from build123d import *

# Parameters (mm, degrees)
SKETCH_1_R          = 1.5
EXTRUDE_1_DEPTH     = 20
SKETCH_2_R          = 2.5
EXTRUDE_2_DEPTH     = 3
CUT_EXTRUDE_1_DEPTH = 1.5
CHAMFER_1_SIZE      = 0.5


with BuildPart() as part:
    # 草图1 → 凸台-拉伸1 (new body)
    with BuildSketch(Plane.XY):
        Circle(SKETCH_1_R)
    extrude(amount=EXTRUDE_1_DEPTH)

    # 草图2 → 凸台-拉伸2 (add)
    with BuildSketch(Plane.XY.offset(20)):
        Circle(SKETCH_2_R)
    extrude(amount=EXTRUDE_2_DEPTH)

    # 草图3 → 切除-拉伸1 (cut)
    with BuildSketch(Plane.XY.offset(23)):
        Polygon((0, 1.803382283), (-1.56177487, 0.901691141), (-1.56177487, -0.901691141), (0, -1.803382283), (1.56177487, -0.901691141), (1.56177487, 0.901691141), align=None)
    extrude(amount=-CUT_EXTRUDE_1_DEPTH, mode=Mode.SUBTRACT)

    # 倒角1
    chamfer_1_edges = [part.edges().sort_by_distance(p)[0] for p in [
        (-1.5, 0, 0),
    ]]
    chamfer(chamfer_1_edges, length=CHAMFER_1_SIZE)


solid = part.part
Check sheet for the modelled part. Datum: model origin and axes. Units: mm. A direction names the side the tool comes from. Coordinates: 2 decimals unless noted, no trailing zeros. Write each loop counter-clockwise with the first axis right and the second up, starting at its lowest first coordinate (ties: lowest second). Pieces come first, ordered by that corner, then holes.
Item 1: Access from +Z, -Z, +X, -X, +Y, -Y to the whole of each face (thin tool, end or side, straight path). Record for faces 1 (the face through (-1.562, 0, 22)), 2 (the face through (2, 0, 23)), 3 (the face through (0, -2, 20)).
Numbers:
face 1: +Z
face 2: +Z, +X, -X, +Y, -Y
face 3: -Z
Item 2: Cross-section at C-C on z = 19. Record the boundary of the cut face in (x, y), then the cut area to 3 significant figures.
Numbers:
outline: circle Ø3 at (0, 0)
area: 7.07 mm2
Item 3: Cross-section at B-B on x = -2. Record the boundary of the cut face in (y, z), then the cut area to 3 significant figures.
Numbers:
outline: (-1.5, 20) - (1.5, 20) - (1.5, 23) - (-1.5, 23) - close
area: 9.00 mm2
Item 4: Cross-section at A-A on y = 0. Record the boundary of the cut face in (x, z).
Numbers:
outline: (-2.5, 20) - (-1.5, 20) - (-1.5, 0.5) - (-1, 0) - (1, 0) - (1.5, 0.5) - (1.5, 20) - (2.5, 20) - (2.5, 23) - (1.56, 23) - (1.56, 21.5) - (-1.56, 21.5) - (-1.56, 23) - (-2.5, 23) - close
Item 5: Scan lines: probe 1 along Z at (x, y) = (-1.9, 0.75); probe 2 along Z at (x, y) = (0.1, -0.7); probe 3 along Y at (x, z) = (1.2, 17). Record each from-to range of solid material in increasing order.
Numbers:
probe 1: z = 20 to 23
probe 2: z = 0 to 21.5
probe 3: y = -0.9 to 0.9
Item 6: Mould release check, pull along X, two halves, no side actions. Record for faces 4 (the face through (0, 0, 0)), 5 (the face through (-0.54, -2.44, 21.48)), 6 (the face through (-0.77, 1.36, 22.26)): released by +X, released by -X, zero draft, split by the parting line, or undercut.
Numbers:
face 4: zero draft
face 5: split by the parting line
face 6: undercut
Item 7: Depth check by flat-ended pin: pin 1 Ø2 at (y, z) = (1.5, 11) entering from -X; pin 2 Ø1.5 at (y, z) = (1.5, 12) entering from +X; pin 3 Ø0.9 at (x, y) = (-0.5, 0.5) entering from +Z. Enter the tip coordinate at first touch or a pass-through.
Numbers:
pin 1: stops at x = -1.41
pin 2: stops at x = 1.3
pin 3: stops at z = 21.5
Item 8: Cross-section at D-D on y = 2.25. Record the boundary of the cut face in (x, z), then the cut area to 3 significant figures.
Numbers:
outline: (-1.09, 20) - (1.09, 20) - (1.09, 23) - (-1.09, 23) - close
area: 6.54 mm2
